Could you check a few things on this drawing? It's one solid part, dimensions in mm from its lowest x, y, z. A direction names the side the tool comes from. Give positions to 0.01 mm unless a question says otherwise; leave off trailing zeros. Write each loop counter-clockwise with the first axis right and the second up, starting at its lowest first coordinate (ties: lowest second). Pieces come first, ordered by that corner, then holes.
1. On a 3-axis mill with a long thin cutter (end or side, diameter ignored), from which of +Z, -Z, +X, -X, +Y, -Y can I reach the whole of each face in a straight line? I mean the marked faces 4, 5, 6, 7 and 8. Say none if no direction works.
2. Suppose I cut it at B-B (x = 8). Please give me the cut outline in (y, z).
3. If I drill on probe 1 along Z at (x, y) = (8, 6.65); probe 2 along Y at (x, z) = (9.5, 3.3); probe 3 along X at (y, z) = (6.25, 13.5), over which ranges is the centre line in solid material (lowest first)?
4. I'm going to push flat-ended pins straight in: pin 1 (2.5 mm diameter, centred on x = 9, y = 3.5, fed in from +Z); pin 2 (8 mm diameter, centred on x = 8, z = 13.5, fed in from -Y); pin 3 (2 mm diameter, centred on y = 3, z = 3, fed in from +X). Where does each tip first touch, or does it pass through?
5. Suppose I cut it at A-A (y = 2). Please give me the cut outline in (x, z).
6. Suppose I cut it at C-C (z = 18.5). Please give me the cut outline in (x, y) (1 decimal).
7. Thinking about a two-plate mould opening in X: for the marked faces 1, 2 and 3, which applies, pulls with the +X half, pulls with the -X half, needs draft (parallel to the pull), parting line crosses it, or undercut?
8. Suppose I cut it at D-D (y = 3). Please give me the cut outline in (x, z).
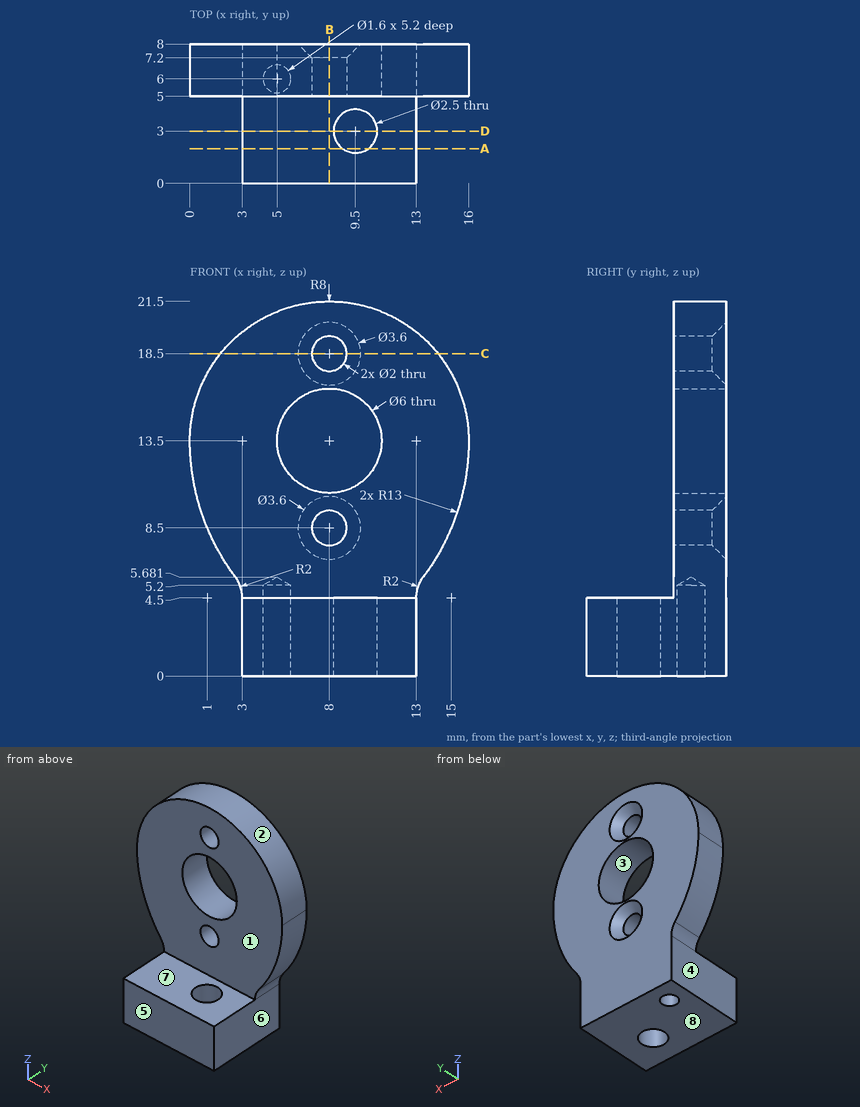
Checks:
1. face 4: -Z, -X, +Y, -Y
1. face 5: +Z, -Z, +X, -X, -Y
1. face 6: -Z, +X, +Y, -Y
1. face 7: +Z, +X, -X, -Y
1. face 8: -Z, +X, -X, +Y, -Y
2. outline: (0, 0) - (8, 0) - (8, 6.7) - (7.2, 7.5) - (5, 7.5) - (5, 4.5) - (0, 4.5) - close; (5, 9.5) - (7.2, 9.5) - (8, 10.3) - (8, 10.5) - (5, 10.5) - close; (5, 16.5) - (8, 16.5) - (8, 16.7) - (7.2, 17.5) - (5, 17.5) - close; (5, 19.5) - (7.2, 19.5) - (8, 20.3) - (8, 21.5) - (5, 21.5) - close
3. probe 1: z = 0 to 7.5, 9.5 to 10.5, 16.5 to 17.5, 19.5 to 21.5
3. probe 2: y = 0 to 1.75, 4.25 to 8
3. probe 3: x = 0 to 5, 11 to 16
4. pin 1: stops at z = 4.5
4. pin 2: stops at y = 5
4. pin 3: stops at x = 13
5. outline: (3, 0) - (8.75, 0) - (8.75, 4.5) - (3, 4.5) - close; (10.25, 0) - (13, 0) - (13, 4.5) - (10.25, 4.5) - close
6. outline: (1.8, 5) - (7, 5) - (7, 7.2) - (6.2, 8) - (1.8, 8) - close; (9, 5) - (14.2, 5) - (14.2, 8) - (9.8, 8) - (9, 7.2) - close
7. face 1: needs draft
7. face 2: parting line crosses it
7. face 3: undercut
8. outline: (3, 0) - (8.25, 0) - (8.25, 4.5) - (3, 4.5) - close; (10.75, 0) - (13, 0) - (13, 4.5) - (10.75, 4.5) - close
